Input: part model. Units: mm. Frame: model coordinates. A direction names the side the tool comes from. Give positions to 0.01 mm unless a question says otherwise; leave off trailing zeros. Loops run counter-clockwise (first coordinate to the right, second up) from the corner with the lowest first, then second, coordinate; pieces in that order, holes last. Notation, with made-up numbers: (-5.5, 50.5) - (48.5, 50.5) arc R32 ccw to (48.5, 78.5) - close; hole circle Ø3 at (59.25, 53.5). An arc over 180 degrees is marked (long way). Answer as a JSON object with one key per item and string values. Group by question number.
(1) Pin query (flat end, axial travel): P1, Ø13.5, axis at x = 2.5, y = 3.5, coming from the +Z side; P2, Ø4, axis at y = 10, z = 22.5, coming from the +X side; P3, Ø2, axis at y = 26, z = 13.5, coming from the -X side. Return the tip coordinate at first contact, or that it passes through.
(2) Mould query, pull axis Y, two halves, no side actions, for faces 1 (the flat face through (0.547, -31.954, 39.44)), 2 (the flat face through (0.505, -29.176, 40.961)), 3 (the flat face through (-0.505, 29.176, 40.961)), 4 (the flat face through (0, 0, 0)). Classes: +Y half, -Y half, draft (parallel to the pull), parting line (faces both ways), or undercut.
(3) Material intervals for L1, parallel to Y at x = -17.5, z = 16.5; L2, parallel to X at y = -25, z = 63.5; L3, parallel to Y at x = -33, z = 64, sorted ascending.
(4) Section query A-A (z = 27.5). Return loops of the section in (x, y), plus the area to 3 significant figures.
(5) Section query B-B (y = -11.5). Return loops of the section in (x, z).
(6) Access query for faces 5 (the flat face through (-31.954, -0.547, 39.44)), 6 (the flat face through (29.176, 0.505, 40.961)). Directions: +Z, -Z, +X, -X, +Y, -Y. A direction counts if a zero-diameter tool reaches every point of the face in a straight line with its end or side. Return the directions, or none.
(7) Section query D-D (z = 40). Return loops of the section in (x, y).
Autodesk Fusion 360 part; units mm, degrees
sketch "스케치1" plane through (0, 0, 0) normal (0, 0, 1) x (1, 0, 0)
  line L0 (-25, 25) -> (25, 25)
  line L1 (25, 25) -> (25, -25)
  line L2 (25, -25) -> (-25, -25)
  line L3 (-25, -25) -> (-25, 25)
sketch "스케치2" plane through (0, 0, 0) normal (0, 0, 1) x (1, 0, 0)
  line L0 (-54.7462, 3.4053) -> (-38.8986, -3.0124)
  line L1 (-38.8986, -3.0124) -> (-94.0377, -2.8814)
  line L2 (-94.0377, -2.8814) -> (-70, 5)
  line L3 (-70, 5) -> (-70, -25)
  line L4 (-70, -25) -> (-54.7462, 3.4053)
extrude "돌출1" add sketch "스케치1" along normal blind 30 draft 10
extrude "돌출2" add 1 faces at (-10.0966, 10.0966, 30) along direction (0, 0, 1) blind 50 draft 10
shell "쉘1" thickness 3 removed faces 1 at (-13.0354, 13.0354, 80)
Recorded:
{
 "1": {"P1": "stops at z = 3", "P2": "stops at x = 29.32", "P3": "stops at x = -27.56"},
 "2": {"face 1": "-Y half", "face 2": "undercut", "face 3": "undercut", "face 4": "draft"},
 "3": {"L1": "y = -27.91 to -24.86, 24.86 to 27.91", "L2": "x = -36.2 to -33.15, 33.15 to 36.2", "L3": "y = -36.28 to -33.24, 33.24 to 36.28"},
 "4": {"outline": "(-29.85, -29.85) - (29.85, -29.85) - (29.85, 29.85) - (-29.85, 29.85) - close; hole (-26.8, -26.8) - (26.8, -26.8) - (26.8, 26.8) - (-26.8, 26.8) - close", "area": "690 mm^2"},
 "5": {"outline": "(-39.11, 80) - (-25, 0) - (25, 0) - (39.11, 80) - (36.06, 80) - (22.48, 3) - (-22.48, 3) - (-36.06, 80) - close"},
 "6": {"face 5": "-Z, -X, +Y, -Y", "face 6": "+Z"},
 "7": {"outline": "(-32.05, -32.05) - (32.05, -32.05) - (32.05, 32.05) - (-32.05, 32.05) - close; hole (-29.01, -29.01) - (29.01, -29.01) - (29.01, 29.01) - (-29.01, 29.01) - close"}
}
